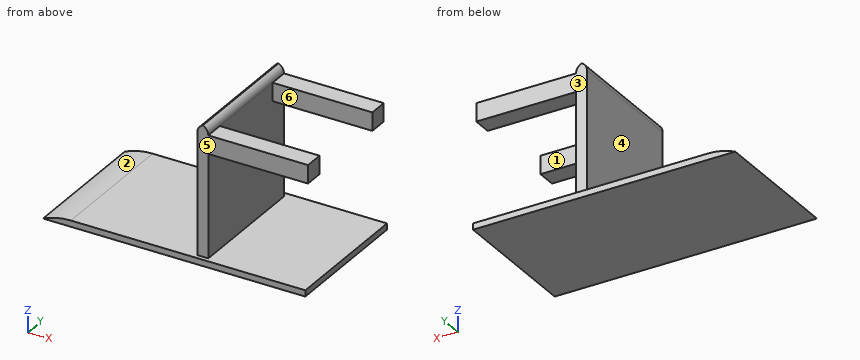
from build123d import *

# Parameters (mm, degrees)
F0_W        = 68.1868493557
F0_H        = 55.5541068316
F1_DEPTH    = 2.54
F2_T1_DEPTH = 112.6971628242
F3_W        = 4.4784088386
F3_H        = 51.4798170188
F4_DEPTH    = 53.34
F5_T1_DEPTH = 69.8761243641
F6_W        = 7.8073056648
F6_H        = 7.4690097984
F6_W_2      = 7.7111199498
F7_DEPTH    = 40.894
F8_DEPTH    = 39.37


# Not quite as in the source:
# - a fillet or chamfer that OpenCascade refuses, or shapes differently, is made with other operations: its cross-section is extruded or revolved along the edge and cut away or added


with BuildPart() as f1:
    # F0 (on Top) → F1 (new body)
    with BuildSketch(Plane.XY):
        with Locations((-34.0934246778, 27.7770534158)):
            Rectangle(F0_W, F0_H)
    extrude(amount=F1_DEPTH)

    # F2: fillet of radius 26.9812507731 on 1 edges, made by hand

    # F2_s2 → F2_t1 (cut)
    with BuildSketch(Plane.XZ.offset(-84.1256348279)):
        with BuildLine():
            ThreePointArc((-68.1868493557, 0), (-62.6119710245, 1.8973464712), (-56.7582381572, 2.54))
            Line((-56.7582381572, 2.54), (-68.1868493557, 2.54))
            Line((-68.1868493557, 2.54), (-68.1868493557, 0))
        make_face()
    extrude(amount=F2_T1_DEPTH, mode=Mode.SUBTRACT)

    # F3 (on face) → F4 (join)
    with BuildSketch(Plane.XY.offset(2.54)):
        with Locations((-3.760119027, 27.5797095965)):
            Rectangle(F3_W, F3_H)
    extrude(amount=F4_DEPTH)

    # F5: fillet of radius 3.6792614691 on 2 edges, made by hand

    # F5_s2 → F5_t1 (cut)
    with BuildSketch(Plane.XZ.offset(-62.5177717785)):
        with BuildLine():
            ThreePointArc((-1.5209146077, 52.2007385309), (-2.5985453422, 54.8023692655), (-5.2001760767, 55.88))
            Line((-5.2001760767, 55.88), (-1.5209146077, 55.88))
            Line((-1.5209146077, 55.88), (-1.5209146077, 52.2007385309))
        make_face()
        with BuildLine():
            ThreePointArc((-5.9993234463, 52.2007385309), (-4.9216927118, 54.8023692655), (-2.3200619772, 55.88))
            Line((-2.3200619772, 55.88), (-5.9993234463, 55.88))
            Line((-5.9993234463, 55.88), (-5.9993234463, 52.2007385309))
        make_face()
    extrude(amount=F5_T1_DEPTH, mode=Mode.SUBTRACT)

    # F6 (on face) → F7 (join)
    with BuildSketch(Plane.YZ.offset(-1.5209146077)):
        with Locations((5.7434539194, 48.4662336318)):
            Rectangle(F6_W, F6_H)
        with Locations((49.464058131, 48.4662336318)):
            Rectangle(F6_W_2, F6_H)
    extrude(amount=F7_DEPTH)

    # F8 (add): a face of the model
    f8_faces = [f1.faces().sort_by_distance(p)[0] for p in [
        (0, 27.7770534158, 1.27),
    ]]
    extrude(f8_faces, amount=F8_DEPTH)


solid = f1.part
Can you work these out from the model? Positions are in its coordinate system, mm. Face numbers are marked on the shaded views. A direction names the side the tool comes from. Coordinates: 2 decimals unless noted, no trailing zeros. Order: outer loops, then holes, each group sorted by start corner. A loop starts at its lowest first (then second) coordinate and runs counter-clockwise, first axis right, second up. Notation, with made-up numbers: (-32, -31.75) - (15, -31.75) arc R28 cw to (15, 6.25) - close; hole circle Ø9 at (70, 9.5). An arc over 180 degrees is marked (long way). Answer as a JSON object with one key per item and string values. Group by question number.
Q1. We'd pull the mould along Y, two halves only. Please class the marked faces 3, 4, 5 and 6: +Y half, -Y half, draft (parallel to the pull), parting line (faces both ways), or undercut.
Q2. I need wall thicknesses on line 1 (Z direction, x = 26.5, y = 15.5); line 2 (X direction, y = 48.5, z = 29.5); line 3 (X direction, y = 3.5, z = 53). Which ranges of each line are inside material? Lowest first, please. Write a range as from..to.
Q3. Imagine slicing it at C-C (z = 48). Please give me the cut outline in (x, y), and give its area (3 significant figures).
Q4. Imagine slicing it at A-A (x = 8.5). Please give me the cut outline in (y, z), and give its area (3 significant figures).
Q5. Imagine slicing it at B-B (y = 17). Please give me the cut outline in (x, z).
Q6. Imagine slicing it at D-D (y = 7). Please give me the cut outline in (x, z).
Q7. Will these pins go through, and if not, where does the flat tip stop? P1, Ø3, axis at y = 42, z = 49.5, coming from the -X side; P2, Ø2.5, axis at x = 18, y = 6, coming from the +Z side; P3, Ø3, axis at y = 31.5, z = 1, coming from the +X side; P4, Ø22.5, axis at x = 15, z = 32.5, coming from the +Y side.
Q8. On a 3-axis mill with a long thin cutter (end or side, diameter ignored), from which of +Z, -Z, +X, -X, +Y, -Y can I reach the whole of each face in a straight line? I mean the marked faces 1 and 2. Say none if no direction works.
Determined:
{
 "1": {"face 3": "+Y half", "face 4": "draft", "face 5": "-Y half", "face 6": "undercut"},
 "2": {"line 1": "z = 0..2.54", "line 2": "x = -6..-1.52", "line 3": "x = -5.91..-1.61"},
 "3": {"outline": "(-6, 1.84) - (39.37, 1.84) - (39.37, 9.65) - (-1.52, 9.65) - (-1.52, 45.61) - (39.37, 45.61) - (39.37, 53.32) - (-6, 53.32) - close", "area": "865 mm2"},
 "4": {"outline": "(0, 0) - (55.55, 0) - (55.55, 2.54) - (0, 2.54) - close; (1.84, 44.73) - (9.65, 44.73) - (9.65, 52.2) - (1.84, 52.2) - close; (45.61, 44.73) - (53.32, 44.73) - (53.32, 52.2) - (45.61, 52.2) - close", "area": "257 mm2"},
 "5": {"outline": "(-68.19, 0) - (39.37, 0) - (39.37, 2.54) - (-1.52, 2.54) - (-1.52, 52.2) arc R3.68 ccw to (-3.76, 55.59) arc R3.68 ccw to (-6, 52.2) - (-6, 2.54) - (-56.76, 2.54) arc R26.98 ccw to start"},
 "6": {"outline": "(-68.19, 0) - (39.37, 0) - (39.37, 2.54) - (-1.52, 2.54) - (-1.52, 44.73) - (39.37, 44.73) - (39.37, 52.2) - (-1.52, 52.2) arc R3.68 ccw to (-3.76, 55.59) arc R3.68 ccw to (-6, 52.2) - (-6, 2.54) - (-56.76, 2.54) arc R26.98 ccw to start"},
 "7": {"P1": "stops at x = -6", "P2": "stops at z = 52.2", "P3": "stops at x = 39.37", "P4": "passes through"},
 "8": {"face 1": "+Z, +X", "face 2": "+Z, -X, +Y, -Y"}
}
